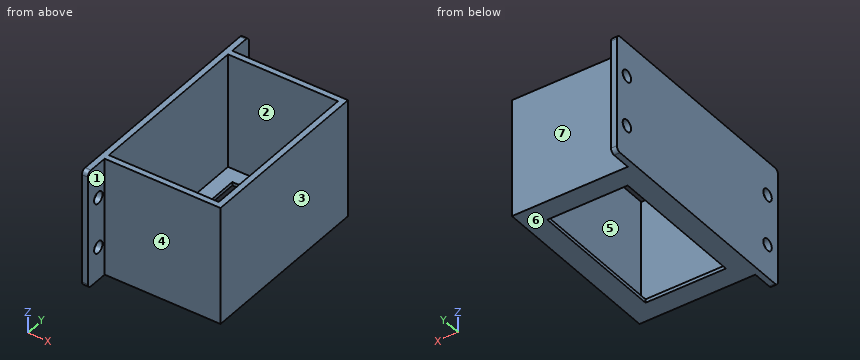
Autodesk Fusion 360 part; units mm, degrees
sketch "Sketch1" plane through (0, 0, 0) normal (0, 0, 1) x (1, 0, 0)
  line L0 (0, 0) -> (27.2, 0)
  line L1 (27.2, 0) -> (27.2, 46.8)
  line L2 (27.2, 46.8) -> (0, 46.8)
  line L3 (0, 46.8) -> (0, 0)
  line L4 (-5, 51.8) -> (-5, -5)
  line L5 (-5, -5) -> (32.2, -5)
  line L6 (32.2, -5) -> (32.2, 51.8)
  line L7 (32.2, 51.8) -> (-5, 51.8)
  line L8 (-7, 53.8) -> (-7, -7)
  line L9 (-7, -7) -> (34.2, -7)
  line L10 (34.2, -7) -> (34.2, 53.8)
  line L11 (34.2, 53.8) -> (-7, 53.8)
  dimension "d1" = 27.2
  dimension "d2" = 46.8
  dimension "d3" = 5
  dimension "d4" = 7
extrude "Extrude1" add sketch "Sketch1" along normal blind 1.2 contours L4 L5 L6 L7
extrude "Extrude2" add sketch "Sketch1" along normal blind 40 contours L8 L9 L10 L11
sketch "Sketch2" plane through (0, 0, 40) normal (0, 0, 1) x (-1, 0, 0)
  line L0 (5, -51.8) -> (-32.2, -51.8)
  line L1 (-32.2, -51.8) -> (-32.2, 5)
  line L2 (-32.2, 5) -> (5, 5)
  line L3 (5, 5) -> (5, -51.8)
  line L4 (-34.2, -53.8) -> (7, -53.8)
  line L5 (7, -53.8) -> (7, 7)
  line L6 (7, 7) -> (-34.2, 7)
  line L7 (-34.2, 7) -> (-34.2, -53.8)
  line L8 (7, -53.8) -> (10.9437, -53.8)
  line L9 (10.9437, -53.8) -> (10.9437, 7)
  line L10 (10.9437, 7) -> (7, 7)
  line L11 (7, 7) -> (7, -53.8)
sketch "Sketch3" plane through (0, -7, 0) normal (0, -1, 0) x (1, 0, 0)
  line L0 (-7, 0) -> (34.2, 0)
  line L1 (34.2, 0) -> (34.2, 40)
  line L2 (34.2, 40) -> (-7, 40)
  line L3 (-7, 40) -> (-7, 0)
  line L4 (-7, 0) -> (-5, 0)
  line L5 (-5, 0) -> (-5, 40)
  line L6 (-5, 40) -> (-7, 40)
  line L7 (-7, 40) -> (-7, 0)
  dimension "d9" = 2
extrude "Extrude3" add sketch "Sketch3" along normal blind 8 contours L0 L2 L3 L4 L5 L6 L7
sketch "Sketch4" plane through (0, 53.8, 0) normal (0, 1, 0) x (-1, 0, 0)
  line L0 (-34.2, 0) -> (7, 0)
  line L1 (7, 0) -> (7, 40)
  line L2 (7, 40) -> (-34.2, 40)
  line L3 (-34.2, 40) -> (-34.2, 0)
  line L4 (7, 0) -> (5, 0)
  line L5 (5, 0) -> (5, 40)
  line L6 (5, 40) -> (7, 40)
  line L7 (7, 40) -> (7, 0)
  dimension "d12" = 2
extrude "Extrude4" add sketch "Sketch4" along normal blind 8 contours L0 L1 L2 L4 L5 L6 L7
fillet "Fillet1" radius 1.5 4 edges at (-6, -15, 40) (-6, 61.8, 40) (-6, 61.8, 0) (-6, -15, 0)
sketch "Sketch5" plane through (-5, 0, 0) normal (1, 0, 0) x (0, 1, 0)
  arc A0 (60.3, 0) -> (61.8, 1.5) centre (60.3, 1.5) ccw
  line L0 (61.8, 1.5) -> (61.8, 38.5)
  arc A1 (61.8, 38.5) -> (60.3, 40) centre (60.3, 38.5) ccw
  line L1 (60.3, 40) -> (53.8, 40)
  line L2 (53.8, 40) -> (53.8, 0)
  line L3 (53.8, 0) -> (60.3, 0)
  line L4 (61.8, 11.3134) -> (-15, 11.3134) construction
  line L5 (61.8, 28.4248) -> (-15, 28.4248) construction
  line L6 (57.05, 0) -> (57.05, 40) construction
  line L7 (-10, 0) -> (-10, 40) construction
  circle A2 centre (57.05, 11.3134) radius 2
  circle A3 centre (57.05, 28.4248) radius 2
  circle A4 centre (-10, 11.3134) radius 2
  circle A5 centre (-10, 28.4248) radius 2
  dimension "d17" = 4
  dimension "d18" = 4
  dimension "d19" = 4
  dimension "d20" = 4
extrude "Extrude5" cut sketch "Sketch5" against normal blind 4 contours A2 | A3 | A4 | A5
equation "d4 = 12 mm - 5 mm"
Part model, mm, in its own coordinate system. Face numbers are marked on the shaded views. A direction names the side the tool comes from. Round coordinates to 2 decimals unless told otherwise and drop trailing zeros. Order: outer loops, then holes, each group sorted by start corner. A loop starts at its lowest first (then second) coordinate and runs counter-clockwise, first axis right, second up. Notation, with made-up numbers: M 88.5,74 L 105.5,74 A23 ccw 105.5,92 Z; hole C -22.5,-0.75 d5. An arc over 180 degrees is marked long. Answer in a Markdown table with one row per item. Add a question column.
Q1. Cut at B-B on y = 57.05. Give the cut face in (x, z).
Q2. 3-axis set-ups, long thin cutter, end or side, ignore diameter. For the marked faces 1, 2 and 3: which of +Z, -Z, +X, -X, +Y, -Y reach the whole face in a straight line?
Q3. Pin check, flat tips, straight feed: pin 1 (8 mm diameter, centred on x = 4.5, z = 26, fed in from -Y); pin 2 (2.5 mm diameter, centred on y = 56.5, z = 19.5, fed in from +X); pin 3 (11 mm diameter, centred on x = 19.5, z = 15, fed in from +Y); pin 4 (3.5 mm diameter, centred on y = 57.05, z = 28.42, fed in from -X). Stop position of each tip, or through.
Q4. Cut at D-D on x = 31. Give the cut face in (y, z), and give its area (3 significant figures).
Q5. Mould opens along Y. For the marked faces 4, 5, 6 and 7 say: +Y half, -Y half, draft (parallel to the pull), parting line (faces both ways), or undercut.
Q6. Cut at A-A on x = 25.5. Give the cut face in (y, z), and give its area (3 significant figures).
Q7. Cut at C-C on z = 24. Give the cut face in (x, y), and give its area (3 significant figures).
Q8. Wall check: L1, parallel to Z at x = -6, y = -10; L2, parallel to Y at x = 31, z = 10.5; L3, parallel to X at y = 4, z = 12. Give the ranges that are in metal, low to high. Write a range as from..to.
Established:
| question | item | result |
|---|---|---|
| 1 | outline | M -7,0 L -5,0 L -5,9.31 L -7,9.31 Z; M -7,13.31 L -5,13.31 L -5,26.42 L -7,26.42 Z; M -7,30.42 L -5,30.42 L -5,40 L -7,40 Z |
| 2 | face 1 | +Z, -Z, +X, -Y |
| 2 | face 2 | +Z |
| 2 | face 3 | +Z, -Z, +X, +Y, -Y |
| 3 | pin 1 | stops at y = -7 |
| 3 | pin 2 | stops at x = -5 |
| 3 | pin 3 | stops at y = 53.8 |
| 3 | pin 4 | passes through |
| 4 | outline | M -7,0 L 53.8,0 L 53.8,40 L 51.8,40 L 51.8,1.2 L -5,1.2 L -5,40 L -7,40 Z |
| 4 | area | 228 mm2 |
| 5 | face 4 | -Y half |
| 5 | face 5 | undercut |
| 5 | face 6 | draft |
| 5 | face 7 | +Y half |
| 6 | outline | M -7,0 L 0,0 L 0,1.2 L -5,1.2 L -5,40 L -7,40 Z; M 46.8,0 L 53.8,0 L 53.8,40 L 51.8,40 L 51.8,1.2 L 46.8,1.2 Z |
| 6 | area | 172 mm2 |
| 7 | outline | M -7,-15 L -5,-15 L -5,-7 L 34.2,-7 L 34.2,53.8 L -5,53.8 L -5,61.8 L -7,61.8 Z; hole M -5,-5 L 32.2,-5 L 32.2,51.8 L -5,51.8 Z |
| 7 | area | 424 mm2 |
| 8 | L1 | z = 0..9.31, 13.31..26.42, 30.42..40 |
| 8 | L2 | y = -7..-5, 51.8..53.8 |
| 8 | L3 | x = -7..-5, 32.2..34.2 |
